For this review, take the finished solid that the model builds, in its own axes (mm). A direction names the side the tool comes from. Give positions to 0.01 mm unless a question says otherwise; leave off trailing zeros. Write each loop counter-clockwise with the first axis right and the second up, starting at its lowest first coordinate (ties: lowest second). Pieces come first, ordered by that corner, then holes.
Q1. Insertion check: P1, Ø7.5, axis at x = -8, z = 20, coming from the -Y side; P2, Ø5.5, axis at x = 8, z = 22.5, coming from the +Y side; P3, Ø10, axis at y = -10, z = 7, coming from the +X side; P4, Ø2.5, axis at x = 15, y = 0, coming from the -Z side. Each pin has a flat end and moves straight along its axis. Give the tip position at first contact, or say it passes through.
Q2. Machinability: for faces 4 (the cylindrical face through (14, 0, 2)), 5 (the cylindrical face through (0, 4.5, 16.3)), 6 (the flat face through (-4, -3.25, 16)), 7 (the flat face through (7, -1.25, 16)), which of the approach directions +Z, -Z, +X, -X, +Y, -Y give a long, thin tool a straight path to every point of the face, cutting with its end or side? Answer none if there is none.
Q3. We need section B-B (z = 17). Write out the cut boundary in (x, y).
Q4. We need section C-C (y = 0). Write out the cut boundary in (x, z), then the cut area to 3 significant figures.
Q5. Mouldability with a two-part tool opening along Y and no side actions: class faces 1 (the flat face through (4, -3.25, 16)), 2 (the flat face through (0, 0, 4)), 3 (the flat face through (5.269, -6, 11)) as released by +Y, released by -Y, zero draft, split by the parting line, or undercut.
Q6. For line 1 (Y direction, x = 0, z = 1.4); line 2 (X direction, y = -1, z = 13.25); line 3 (X direction, y = 5.5, z = 5.25), list the stretches that pass through material, from the lowest coordinate up.
Q7. We need section A-A (x = 0). Write out the cut boundary in (y, z), then the cut area to 3 significant figures.
Q8. We need section D-D (x = -15). Write out the cut boundary in (y, z), then the cut area to 3 significant figures.
```python
from build123d import *

# Parameters (mm, degrees)
F0_R     = 21
F1_DEPTH = 4
F2_D     = 2
F4_DEPTH = 25
F6_DEPTH = 7


with BuildPart() as f1:
    # F0 (on Top) → F1 (new body)
    with BuildSketch(Plane.XY):
        Circle(F0_R)
    extrude(amount=F1_DEPTH)

    # F2 (through all)
    with Locations(Plane(origin=(0, 0, 0), x_dir=(1, 0, 0), z_dir=(0, 0, -1))):
        with Locations((-15, 0), (0, 9), (0, -9), (15, 0)):
            Hole(F2_D / 2)

    # F3 (on face) → F4 (join)
    with BuildSketch(Plane.XY.offset(4)):
        with BuildLine():
            ThreePointArc((-4.3229041164, 1.25), (-3.8498331493, 2.3299752622), (-3.1124748995, 3.25))
            Line((-3.1124748995, 3.25), (-12.2691742077, 3.25))
            Line((-12.2691742077, 3.25), (-12.2691742077, -3.25))
            Line((-12.2691742077, -3.25), (-3.1124748995, -3.25))
            ThreePointArc((-3.1124748995, -3.25), (-3.8498331493, -2.3299752622), (-4.3229041164, -1.25))
            Line((-4.3229041164, -1.25), (-10.2691742077, -1.25))
            Line((-10.2691742077, -1.25), (-10.2691742077, 1.25))
            Line((-10.2691742077, 1.25), (-4.3229041164, 1.25))
        make_face()
        with BuildLine():
            ThreePointArc((-1.2990381057, 3.25), (0, 3.5), (1.2990381057, 3.25))
            Line((1.2990381057, 3.25), (3.1124748995, 3.25))
            ThreePointArc((3.1124748995, 3.25), (0, 4.5), (-3.1124748995, 3.25))
            Line((-3.1124748995, 3.25), (-1.2990381057, 3.25))
        make_face()
        with BuildLine():
            ThreePointArc((-3.2691742077, 1.25), (-2.4934195265, 2.4561879132), (-1.2990381057, 3.25))
            Line((-1.2990381057, 3.25), (-3.1124748995, 3.25))
            ThreePointArc((-3.1124748995, 3.25), (-3.8498331493, 2.3299752622), (-4.3229041164, 1.25))
            Line((-4.3229041164, 1.25), (-3.2691742077, 1.25))
        make_face()
        with BuildLine():
            Line((-3.1124748995, -3.25), (-1.2990381057, -3.25))
            ThreePointArc((-1.2990381057, -3.25), (-2.4934195265, -2.4561879132), (-3.2691742077, -1.25))
            Line((-3.2691742077, -1.25), (-4.3229041164, -1.25))
            ThreePointArc((-4.3229041164, -1.25), (-3.8498331493, -2.3299752622), (-3.1124748995, -3.25))
        make_face()
        with BuildLine():
            Line((3.1124748995, -3.25), (1.2990381057, -3.25))
            ThreePointArc((1.2990381057, -3.25), (0, -3.5), (-1.2990381057, -3.25))
            Line((-1.2990381057, -3.25), (-3.1124748995, -3.25))
            ThreePointArc((-3.1124748995, -3.25), (0, -4.5), (3.1124748995, -3.25))
        make_face()
        with BuildLine():
            Line((4.3229041164, -1.25), (3.2691742077, -1.25))
            ThreePointArc((3.2691742077, -1.25), (2.4934195265, -2.4561879132), (1.2990381057, -3.25))
            Line((1.2990381057, -3.25), (3.1124748995, -3.25))
            ThreePointArc((3.1124748995, -3.25), (3.8498331493, -2.3299752622), (4.3229041164, -1.25))
        make_face()
        with BuildLine():
            ThreePointArc((1.2990381057, 3.25), (2.4934195265, 2.4561879132), (3.2691742077, 1.25))
            Line((3.2691742077, 1.25), (4.3229041164, 1.25))
            ThreePointArc((4.3229041164, 1.25), (3.8498331493, 2.3299752622), (3.1124748995, 3.25))
            Line((3.1124748995, 3.25), (1.2990381057, 3.25))
        make_face()
        with BuildLine():
            ThreePointArc((3.1124748995, 3.25), (3.8498331493, 2.3299752622), (4.3229041164, 1.25))
            Line((4.3229041164, 1.25), (10.2691742077, 1.25))
            Line((10.2691742077, 1.25), (10.2691742077, -1.25))
            Line((10.2691742077, -1.25), (4.3229041164, -1.25))
            ThreePointArc((4.3229041164, -1.25), (3.8498331493, -2.3299752622), (3.1124748995, -3.25))
            Line((3.1124748995, -3.25), (12.2691742077, -3.25))
            Line((12.2691742077, -3.25), (12.2691742077, 3.25))
            Line((12.2691742077, 3.25), (3.1124748995, 3.25))
        make_face()
    extrude(amount=F4_DEPTH)

    # F5 (on face) → F6 (join)
    with BuildSketch(Plane.YZ.offset(12.2691742077)):
        Polygon((-3.25, 4), (-3.25, 29), (-13.25, 4), align=None)
        Polygon((13.25, 4), (3.25, 29), (3.25, 4), align=None)
    extrude(amount=-F6_DEPTH)

    # F7: F1 across plane


with BuildPart() as f1_1:
    add(f1.part)
    add(f1.part.mirror(Plane.YZ))


solid = f1_1.part
```
Computed:
1. P1: stops at y = -8.35
1. P2: stops at y = 6.95
1. P3: stops at x = 20.12
1. P4: stops at z = 0
2. face 4: +Z, -Z
2. face 5: +Z, +Y
2. face 6: +Z, -Y
2. face 7: +Z
3. outline: (-12.27, -8.05) - (-5.27, -8.05) - (-5.27, -3.25) - (-3.11, -3.25) arc R4.5 ccw to (3.11, -3.25) - (5.27, -3.25) - (5.27, -8.05) - (12.27, -8.05) - (12.27, 8.05) - (5.27, 8.05) - (5.27, 3.25) - (3.11, 3.25) arc R4.5 ccw to (-3.11, 3.25) - (-5.27, 3.25) - (-5.27, 8.05) - (-12.27, 8.05) - close; hole (-10.27, -1.25) - (-3.27, -1.25) arc R3.5 ccw to (3.27, -1.25) - (10.27, -1.25) - (10.27, 1.25) - (3.27, 1.25) arc R3.5 ccw to (-3.27, 1.25) - (-10.27, 1.25) - close
4. outline: (-21, 0) - (-16, 0) - (-16, 4) - (-21, 4) - close; (-14, 0) - (14, 0) - (14, 4) - (12.27, 4) - (12.27, 29) - (10.27, 29) - (10.27, 4) - (-10.27, 4) - (-10.27, 29) - (-12.27, 29) - (-12.27, 4) - (-14, 4) - close; (16, 0) - (21, 0) - (21, 4) - (16, 4) - close
4. area: 252 mm2
5. face 1: released by -Y
5. face 2: undercut
5. face 3: zero draft
6. line 1: y = -21 to -10, -8 to 8, 10 to 21
6. line 2: x = -12.27 to -10.27, 10.27 to 12.27
6. line 3: x = -12.27 to -5.27, 5.27 to 12.27
7. outline: (-21, 0) - (-10, 0) - (-10, 4) - (-21, 4) - close; (-8, 0) - (8, 0) - (8, 4) - (4.5, 4) - (4.5, 29) - (3.5, 29) - (3.5, 4) - (-3.5, 4) - (-3.5, 29) - (-4.5, 29) - (-4.5, 4) - (-8, 4) - close; (10, 0) - (21, 0) - (21, 4) - (10, 4) - close
7. area: 202 mm2
8. outline: (-14.7, 0) - (-1, 0) - (-1, 4) - (-14.7, 4) - close; (1, 0) - (14.7, 0) - (14.7, 4) - (1, 4) - close
8. area: 110 mm2
